from build123d import *

# Parameters (mm, degrees)
SKETCH1_R           = 2.5
BOSS_EXTRUDE1_DEPTH = 4.5
SKETCH2_W           = 53
SKETCH2_H           = 33
SKETCH2_R           = 12
SKETCH2_R_2         = 2.5
CUT_EXTRUDE2_DEPTH  = 10
SKETCH2_6_R         = 2
SKETCH2_6_W         = 17
SKETCH2_6_H         = 14
CUT_EXTRUDE3_DEPTH  = 10


with BuildPart() as part:
    # Sketch1 → Boss-Extrude1 (new body)
    with BuildSketch(Plane.XY):
        with BuildLine():
            Line((-367, 123.5), (-186, 123.5))
            ThreePointArc((-186, 123.5), (-183.5, 121), (-181, 123.5))
            Line((-181, 123.5), (-2.5, 123.5))
            ThreePointArc((-2.5, 123.5), (0, 121), (2.5, 123.5))
            Line((2.5, 123.5), (181, 123.5))
            ThreePointArc((181, 123.5), (183.5, 121), (186, 123.5))
            Line((186, 123.5), (367, 123.5))
            Line((367, 123.5), (367, -118.5))
            Line((367, -118.5), (-367, -118.5))
            Line((-367, -118.5), (-367, 123.5))
        make_face()
        with Locations((-355, 2.5)):
            Circle(SKETCH1_R, mode=Mode.SUBTRACT)
        with Locations((-355, 64.25)):
            Circle(SKETCH1_R, mode=Mode.SUBTRACT)
        with Locations((-355, -59.25)):
            Circle(SKETCH1_R, mode=Mode.SUBTRACT)
        with Locations(Location((355, -59.25, 0), (0, 0, 180))):
            Circle(SKETCH1_R, mode=Mode.SUBTRACT)
        with Locations(Location((355, 2.5, 0), (0, 0, 180))):
            Circle(SKETCH1_R, mode=Mode.SUBTRACT)
        with Locations(Location((355, 64.25, 0), (0, 0, 180))):
            Circle(SKETCH1_R, mode=Mode.SUBTRACT)
        with Locations((-183.5, -106.5)):
            Circle(SKETCH1_R, mode=Mode.SUBTRACT)
        with Locations((0, -106.5)):
            Circle(SKETCH1_R, mode=Mode.SUBTRACT)
        with Locations((183.5, -106.5)):
            Circle(SKETCH1_R, mode=Mode.SUBTRACT)
    extrude(amount=BOSS_EXTRUDE1_DEPTH)

    # Sketch2 → Cut-Extrude2 (cut)
    with BuildSketch(Plane.XY.offset(4.5)):
        with Locations((-288.5, 69)):
            Rectangle(SKETCH2_W, SKETCH2_H)
        with Locations((-189.425096945, 73.5)):
            Circle(SKETCH2_R)
        Polygon((195.5, -8.117912133), (171.5, -8.117912133), (153.306947094, -26.117912133), (153.306947094, -50.117912133), (171.5, -68.117912133), (195.5, -68.117912133), (213.693052906, -50.117912133), (213.693052906, -26.117912133), align=None)
        with Locations((-189.425096945, -16.5)):
            Circle(SKETCH2_R)
        with Locations((-189.425096945, -61.5)):
            Circle(SKETCH2_R)
        with Locations((208.5, -13.117912133)):
            Circle(SKETCH2_R_2)
        with Locations((208.5, -63.117912133)):
            Circle(SKETCH2_R_2)
        with Locations((158.5, -63.117912133)):
            Circle(SKETCH2_R_2)
        with Locations((158.5, -13.117912133)):
            Circle(SKETCH2_R_2)
        with Locations((219, -2.617912133)):
            Circle(SKETCH2_R_2)
        with Locations((219, -73.617912133)):
            Circle(SKETCH2_R_2)
        with Locations((148, -2.617912133)):
            Circle(SKETCH2_R_2)
        with Locations((148, -73.617912133)):
            Circle(SKETCH2_R_2)
    extrude(amount=-CUT_EXTRUDE2_DEPTH, mode=Mode.SUBTRACT)

    # Sketch2_6 → Cut-Extrude3 (cut)
    with BuildSketch(Plane.XY.offset(4.5)):
        with Locations((-201.185142567, 28.5)):
            Circle(SKETCH2_6_R)
        with Locations((-177.665051324, 28.5)):
            Circle(SKETCH2_6_R)
        with Locations((-189.425096945, 28.5)):
            Rectangle(SKETCH2_6_W, SKETCH2_6_H)
    extrude(amount=-CUT_EXTRUDE3_DEPTH, mode=Mode.SUBTRACT)


solid = part.part
Can you work these out from the model? Positions are in its coordinate system, mm. A direction names the side the tool comes from. Give positions to 0.01 mm unless a question says otherwise; leave off trailing zeros. Loops run counter-clockwise (first coordinate to the right, second up) from the corner with the lowest first, then second, coordinate; pieces in that order, holes last. Notation, with made-up numbers: (61.5, -4.75) -> (72.5, -4.75) arc R9 ccw to (72.5, 3.25) -> close; hole circle Ø9 at (8, 36). An arc over 180 degrees is marked (long way). Return JSON: item names as keys, results as strings.
Q1. For pin 1 Ø14.5 at (x, y) = (-189.43, 73.5) entering from -Z (3 decimals), with a flat end and sliding along its axis, tell me the tip position at first contact or that it passes through.
Checks:
{"pin 1": "passes through"}
Q2. I want a section at B-B, the plane y = -35. List the corners of the cut face in (x, z) for me, then the cut area to 3 significant figures.
Checks:
{"outline": "(-367, 0) -> (153.31, 0) -> (153.31, 4.5) -> (-367, 4.5) -> close; (213.69, 0) -> (367, 0) -> (367, 4.5) -> (213.69, 4.5) -> close", "area": "3,030 mm2"}
Q3. On a 3-axis mill with a long thin cutter (end or side, diameter ignored), from which of +Z, -Z, +X, -X, +Y, -Y can I reach the whole of each face in a straight line? I mean faces 4 (the face through (204.469, -59.244, 2.282)), 5 (the face through (5, 4, 4.5)). Say none if no direction works.
Checks:
{"face 4": "+Z, -Z", "face 5": "+Z, +X, -X, +Y, -Y"}
Q4. I want a section at C-C, the plane z = 1.4. Count the separate pieces of the cut face and the enclosed holes in it, then the cut area to 3 significant figures.
Checks:
{"separate pieces": "1", "enclosed holes": "25", "area": "171,000 mm2"}
Q5. I want a section at A-A, the plane x = -305.5. List the corners of the cut face in (y, z) for me, then the cut area to 4 significant figures.
Checks:
{"outline": "(-118.5, 0) -> (52.5, 0) -> (52.5, 4.5) -> (-118.5, 4.5) -> close; (85.5, 0) -> (123.5, 0) -> (123.5, 4.5) -> (85.5, 4.5) -> close", "area": "940.5 mm2"}
Q6. We'd pull the mould along Y, two halves only. Please class faces 1 (the face through (-192.026, -73.215, 2.282)), 2 (the face through (162.53, -16.99, 2.28)), 3 (the face through (5, 4, 0)): released by +Y, released by -Y, zero draft, split by the parting line, or undercut.
Checks:
{"face 1": "undercut", "face 2": "undercut", "face 3": "zero draft"}
Q7. I need wall thicknesses on probe 1 along X at (y, z) = (-29.5, 0.25); probe 2 along Y at (x, z) = (-272, 1.5); probe 3 along X at (y, z) = (22.5, 0.85). Which ranges of each line are inside material? Lowest first, please.
Checks:
{"probe 1": "x = -367 to 153.31, 213.69 to 367", "probe 2": "y = -118.5 to 52.5, 85.5 to 123.5", "probe 3": "x = -367 to -197.93, -180.93 to 367"}
